Autodesk Inventor part; units mm, degrees
ref_plane "YZ Plane" through (0, 0, 0) normal (1, 0, 0) x (0, 1, 0)
ref_plane "XZ Plane" through (0, 0, 0) normal (0, 1, 0) x (-1, 0, 0)
ref_plane "XY Plane" through (0, 0, 0) normal (0, 0, 1) x (1, 0, 0)
sketch "Sketch1" plane through (0, 0, 0) normal (0, 1, 0) x (-1, 0, 0)
  line L0 (0.224, 8.425) -> (-0.224, 8.425)
  line L1 (-0.224, 8.425) -> (-0.224, -8.425)
  line L2 (-0.224, -8.425) -> (0.224, -8.425)
  line L3 (0.224, -8.425) -> (0.224, 8.425)
  line L4 (0.224, 8.425) -> (-0.224, -8.425) construction
  line L5 (-0.224, 8.425) -> (0.224, -8.425) construction
  point P0 (0, 0)
  dimension "d0" = 0.448
  dimension "d1" = 16.85
extrude "Plate1" add sketch "Sketch1" along normal blind 0.35
sketch "Sketch2" plane through (0.224, 0.4, 8.5116) normal (0, -0.5, 0.8660254) x (1, 0, 0)
  line L0 (-0.448, 0) -> (0, 0)
  line L1 (0, 0) -> (0, 1.7952)
  line L2 (0, 1.7952) -> (-0.448, 1.7952)
  line L3 (-0.448, 1.7952) -> (-0.448, 0)
edge flange "Flange1" height 2.055 angle 60 thickness 0.35 bend radius 0.1 thickness toward (0, -0.5, 0.8660254) relief tear relief width 0.35 relief depth 0.175 edges at (0, 0.35, 8.425) wall of the first edge with corners at (-0.224, 0.4, 8.5116) (0.224, 0.4, 8.5116) (0.224, 1.9547, 9.4092) (-0.224, 1.9547, 9.4092)
bend "Bend1"
corner "Corner1"
sketch "Sketch3" plane through (0.224, 2.0047, 9.4226) normal (0, 0, 1) x (1, 0, 0)
  line L0 (-0.448, 0) -> (0, 0)
  line L1 (0, 0) -> (0, 1.3479)
  line L2 (0, 1.3479) -> (-0.448, 1.3479)
  line L3 (-0.448, 1.3479) -> (-0.448, 0)
edge flange "Flange2" height 1.4685 angle 30 thickness 0.35 bend radius 0.1 thickness toward (0, 0, 1) relief tear relief width 0.35 relief depth 0.175 edges at (0, 1.9547, 9.4092) wall of the first edge with corners at (-0.224, 2.0047, 9.4226) (0.224, 2.0047, 9.4226) (0.224, 3.3526, 9.4226) (-0.224, 3.3526, 9.4226)
bend "Bend2"
corner "Corner2"
sketch "Sketch4" plane through (0.224, 3.4453, 9.3601) normal (0, 0.9271839, 0.3746066) x (-1, 0, 0)
  line L0 (0.448, 0) -> (0, 0)
  line L1 (0, 0) -> (0, -12.6465)
  line L2 (0, -12.6465) -> (0.448, -12.6465)
  line L3 (0.448, -12.6465) -> (0.448, 0)
edge flange "Flange3" height 12.95 angle 68 thickness 0.35 bend radius 0.1 thickness toward (0, 0.9271839, 0.3746066) relief tear relief width 0.35 relief depth 0.175 edges at (0, 3.3526, 9.4226) wall of the first edge with corners at (-0.224, 3.4453, 9.3601) (0.224, 3.4453, 9.3601) (0.224, 8.1828, -2.3655) (-0.224, 8.1828, -2.3655)
bend "Bend3"
corner "Corner3"
equation "\"d2\" = Thickness"
equation "\"d3\" = BendReliefWidth"
equation "\"d4\" = BendReliefDepth"
equation "\"d5\" = MinimumRemnant"
equation "\"d6\" = TransitionRadius"
equation "\"d9\" = BendRadius"
equation "\"d10\" = CornerReliefSize"
equation "\"d11\" = GapSize"
equation "\"d12\" = JacobiRadiusSize"
equation "\"d13\" = BendReliefWidth"
equation "\"d14\" = BendReliefDepth"
equation "\"d15\" = MinimumRemnant"
equation "\"d16\" = TransitionRadius"
equation "\"d19\" = BendRadius"
equation "\"d20\" = CornerReliefSize"
equation "\"d21\" = GapSize"
equation "\"d22\" = JacobiRadiusSize"
equation "\"d23\" = BendReliefWidth"
equation "\"d24\" = BendReliefDepth"
equation "\"d25\" = MinimumRemnant"
equation "\"d26\" = TransitionRadius"
equation "\"d29\" = BendRadius"
equation "\"d30\" = CornerReliefSize"
equation "\"d31\" = GapSize"
equation "\"d32\" = JacobiRadiusSize"
equation "\"BendReliefWidth\" = Thickness"
equation "\"BendReliefDepth\" = 0.5 * Thickness"
equation "\"CornerReliefSize\" = 4 * Thickness"
equation "\"MinimumRemnant\" = 2 * Thickness"
equation "\"TransitionRadius\" = BendRadius"
equation "\"JacobiRadiusSize\" = BendRadius"
equation "\"GapSize\" = Thickness"
properties part number "RJ45 Even Pins" material "Nickel-Copper Alloy 400"
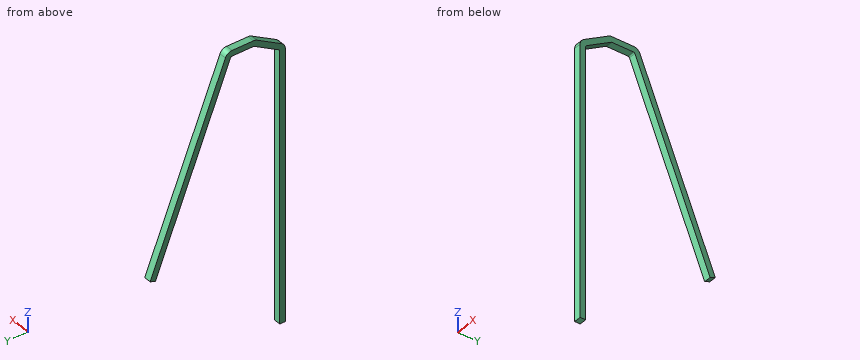
Here's how the part is built. I have some questions about the finished solid (model axes, mm). Coordinates: 2 decimals unless noted, no trailing zeros. Write each loop counter-clockwise with the first axis right and the second up, starting at its lowest first coordinate (ties: lowest second). Pieces come first, ordered by that corner, then holes. Notation, with made-up numbers: (26.5, 8) -> (84.5, 8) arc R34 ccw to (84.5, 39) -> close; hole circle Ø5 at (89.25, 29). An arc over 180 degrees is marked (long way). Use a Markdown table: item, result. Add a question column.
(1) Please list where these lines run through material, in increasing order: line 1 (Y direction, x = -0.1, z = -5); line 2 (Y direction, x = 0.1, z = 6.25); line 3 (Y direction, x = -0.05, z = -1.5).
(2) If we section it at B-B, the plane z = 3: Write out the boundary of the cut face in (x, y).
(3) If we section it at C-C, the plane y = 2.75: Write out the boundary of the cut face in (x, z), and give its area (3 significant figures).
(4) If we section it at D-D, the plane z = -3.75: Write out the boundary of the cut face in (x, y), and give its area (3 significant figures).
Outcome:
| question | item | result |
|---|---|---|
| 1 | line 1 | y = 0 to 0.35 |
| 1 | line 2 | y = 0 to 0.35, 4.7 to 5.08 |
| 1 | line 3 | y = 0 to 0.35, 7.83 to 8.21 |
| 2 | outline | (-0.22, 0) -> (0.22, 0) -> (0.22, 0.35) -> (-0.22, 0.35) -> close; (-0.22, 6.01) -> (0.22, 6.01) -> (0.22, 6.39) -> (-0.22, 6.39) -> close |
| 3 | outline | (-0.22, 9.42) -> (0.22, 9.42) -> (0.22, 9.77) -> (-0.22, 9.77) -> close |
| 3 | area | 0.157 mm^2 |
| 4 | outline | (-0.22, 0) -> (0.22, 0) -> (0.22, 0.35) -> (-0.22, 0.35) -> close |
| 4 | area | 0.157 mm^2 |
